Geometry check sheet. Reference: drawing and pictorial views, mm from the part's lowest x, y, z. A direction names the side the tool comes from. Give positions to 0.01 mm unless a question says otherwise; leave off trailing zeros. Loops run counter-clockwise (first coordinate to the right, second up) from the corner with the lowest first, then second, coordinate; pieces in that order, holes last. Notation, with made-up numbers: (41, -4.5) - (66, -4.5) arc R23 cw to (66, 6.5) - close; hole circle Ø2 at (60, 50). An arc over 180 degrees is marked (long way). Answer in a Markdown table with one row per item. Add a question column.
(1) Set-up check for the marked faces 1 and 2: record each of +Z, -Z, +X, -X, +Y, -Y from which the full face is reachable in a straight line by a thin tool's end or side.
(2) Sectioned sample at B-B on x = 19.05. State how many separate pieces and enclosed holes the cut face has.
(3) Go/stop test with flat-tipped pins: P1, Ø1.6, axis at x = 19, y = 23.5, coming from the +Z side; P2, Ø9, axis at x = 28.67, y = 13.49, coming from the +Z side; P3, Ø1.6, axis at y = 23, z = 17.5, coming from the +X side. Record where each tip stops, or that it passes through.
(4) Sectioned sample at C-C on z = 8. Enter the section's corners in (x, y).
(5) Thickness scan on L1, parallel to Y at x = 19, z = 8.25; L2, parallel to Y at x = 19.05, z = 5.25; L3, parallel to X at y = 10.5, z = 2 (1 decimal). Record the ranges inside material, lowest first.
(6) Draft check along Y on the marked faces 3, 4 and 5. Enter one of: released by +Y, released by -Y, zero draft, split by the parting line, or undercut.
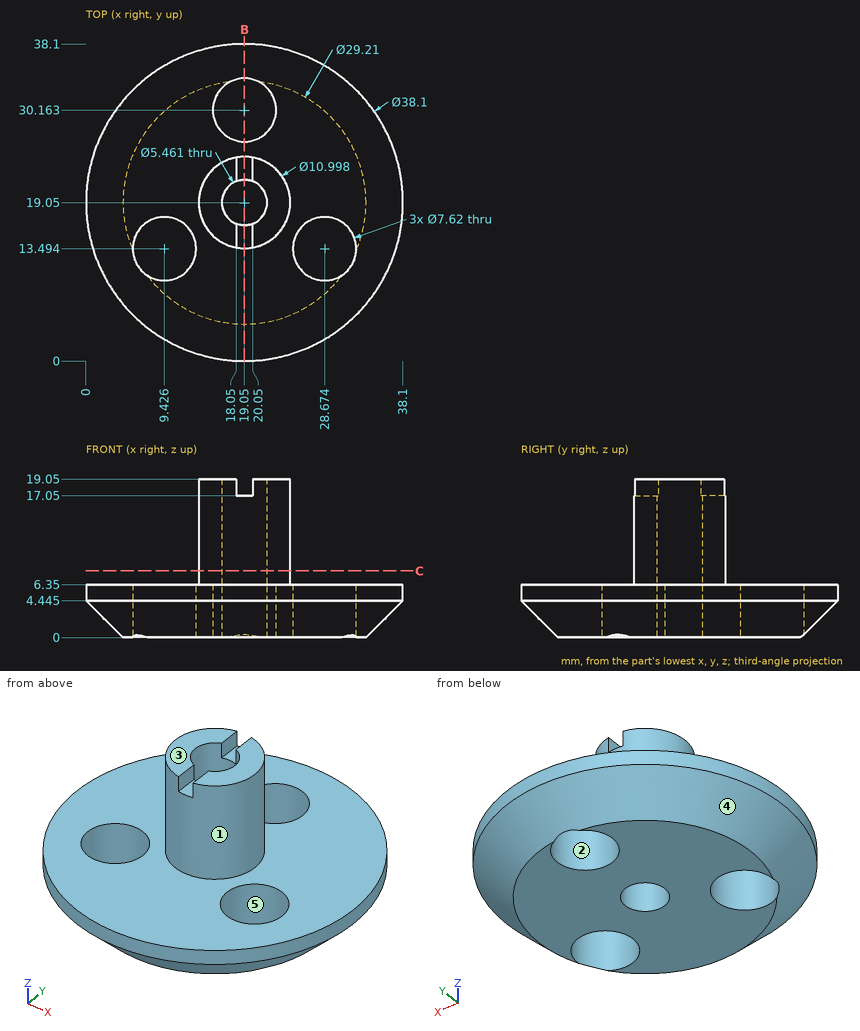
Reply:
| question | item | result |
|---|---|---|
| 1 | face 1 | +Z |
| 1 | face 2 | +Z, -Z |
| 2 | separate pieces | 3 |
| 2 | enclosed holes | 0 |
| 3 | P1 | z = 17.05 |
| 3 | P2 | z = 6.35 |
| 3 | P3 | x = 23.56 |
| 4 | outline | circle Ø11 at (19.05, 19.05); hole circle Ø5.46 at (19.05, 19.05) |
| 5 | L1 | 13.55 to 16.32, 21.78 to 24.55 |
| 5 | L2 | 0 to 16.32, 21.78 to 26.35, 33.97 to 38.1 |
| 5 | L3 | 4.8 to 7.1, 11.8 to 26.3, 31 to 33.3 |
| 6 | face 3 | zero draft |
| 6 | face 4 | split by the parting line |
| 6 | face 5 | undercut |
